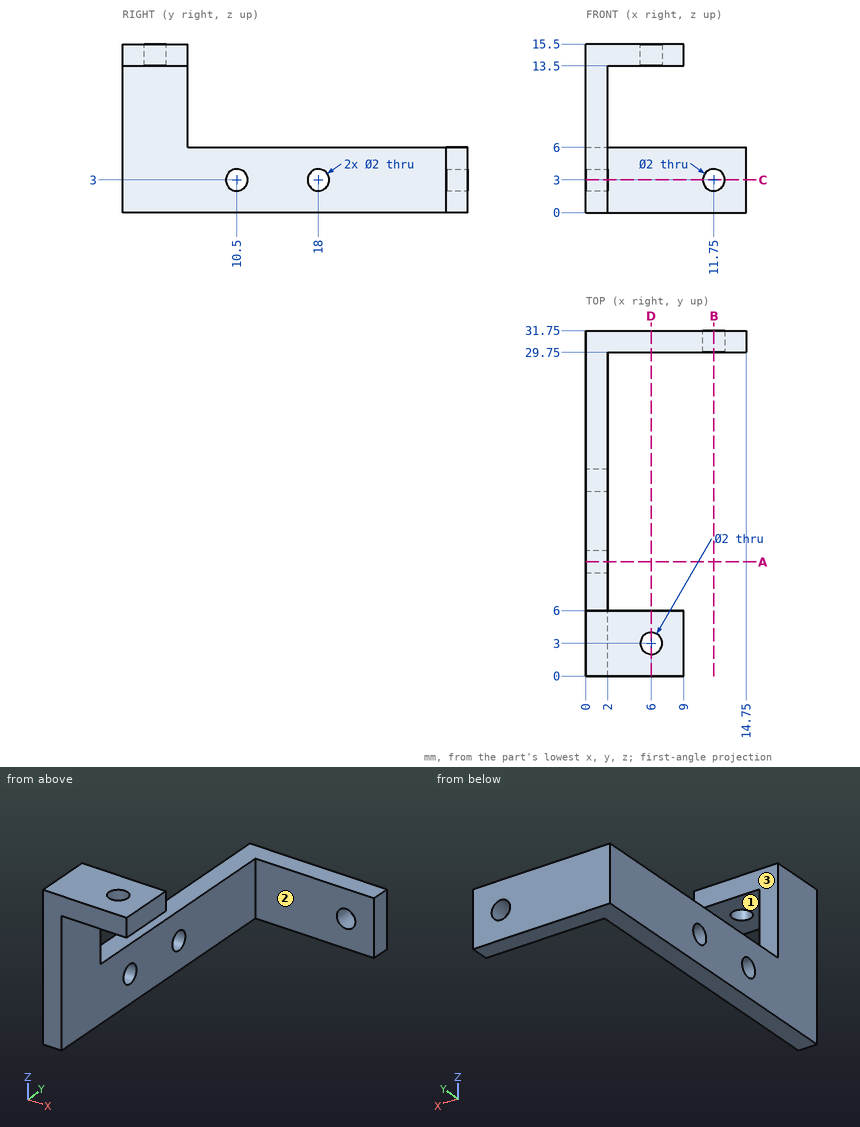
Can you work these out from the drawing? Everything is in mm from the part's minimum corner. A direction names the side the tool comes from. Round coordinates to 2 decimals unless told otherwise and drop trailing zeros. Write each loop counter-clockwise with the first axis right and the second up, starting at its lowest first coordinate (ties: lowest second). Pieces come first, ordered by that corner, then holes. Notation, with made-up numbers: M 87.25,-24 L 114.25,-24 A33 ccw 114.25,5 Z; hole C 66.25,84.5 d2. An arc over 180 degrees is marked long. Use a Markdown table: item, result.
Item 1: For pin 1 Ø1.8 at (x, y) = (7, 4) entering from -Z; pin 2 Ø3 at (x, z) = (6.5, 2) entering from -Y; pin 3 Ø2 at (y, z) = (4.5, 14.5) entering from +X; pin 4 Ø4 at (x, y) = (4, 7) entering from +Z, each with a flat end and sliding along its axis, tell me the tip position at first contact or that it passes through.
Found:
| item | result |
|---|---|
| pin 1 | stops at z = 13.5 |
| pin 2 | stops at y = 29.75 |
| pin 3 | stops at x = 9 |
| pin 4 | stops at z = 15.5 |
Item 2: I want a section at B-B (x = 11.75). List the corners of the cut face in (y, z) for me.
Found:
| item | result |
|---|---|
| outline | M 29.75,0 L 31.75,0 L 31.75,2 L 29.75,2 Z; M 29.75,4 L 31.75,4 L 31.75,6 L 29.75,6 Z |
Item 3: If I drill on line 1 along Z through (x, y) = (0.75, 18); line 2 along X through (y, z) = (2.5, 11); line 3 along Y through (x, z) = (10, 5.75), over which ranges is the centre line in solid material (lowest first)? Write a range as [from, to].
Found:
| item | result |
|---|---|
| line 1 | z = [0, 2], [4, 6] |
| line 2 | x = [0, 2] |
| line 3 | y = [29.75, 31.75] |
Item 4: I want a section at D-D (x = 6). List the corners of the cut face in (y, z) for me.
Found:
| item | result |
|---|---|
| outline | M 0,13.5 L 2,13.5 L 2,15.5 L 0,15.5 Z; M 4,13.5 L 6,13.5 L 6,15.5 L 4,15.5 Z; M 29.75,0 L 31.75,0 L 31.75,6 L 29.75,6 Z |
Item 5: I want a section at C-C (z = 3). List the corners of the cut face in (x, y) for me, and give its area (3 significant figures).
Found:
| item | result |
|---|---|
| outline | M 0,0 L 2,0 L 2,9.5 L 0,9.5 Z; M 0,11.5 L 2,11.5 L 2,17 L 0,17 Z; M 0,19 L 2,19 L 2,29.75 L 10.75,29.75 L 10.75,31.75 L 0,31.75 Z; M 12.75,29.75 L 14.75,29.75 L 14.75,31.75 L 12.75,31.75 Z |
| area | 77.0 mm2 |
Item 6: I want a section at A-A (y = 10.5). List the corners of the cut face in (x, z) for me.
Found:
| item | result |
|---|---|
| outline | M 0,0 L 2,0 L 2,2 L 0,2 Z; M 0,4 L 2,4 L 2,6 L 0,6 Z |
Item 7: Which directions (+Z, -Z, +X, -X, +Y, -Y) give clear straight access to the entire face, cutting with the end or side of a thin tool? Please do the marked faces 1, 2 and 3.
Found:
| item | result |
|---|---|
| face 1 | -Z, +X, +Y, -Y |
| face 2 | +Z, -Z, +X, -Y |
| face 3 | +Z, +X, -X, +Y |
